Model file for the job. Use its own axes, mm. Face numbers are marked on the shaded views. A direction names the side the tool comes from. Give positions to 0.01 mm unless a question says otherwise; leave off trailing zeros. Loops run counter-clockwise (first coordinate to the right, second up) from the corner with the lowest first, then second, coordinate; pieces in that order, holes last. Notation, with made-up numbers: (36, -7.75) -> (65, -7.75) arc R28 cw to (65, 17.25) -> close; hole circle Ø9 at (-29, 17.5). An arc over 180 degrees is marked (long way). Use CSV: the item, a comma, the result in double quotes. Start each with the question number.
(1) 3-axis set-ups, long thin cutter, end or side, ignore diameter. For the marked faces 4, 5, 6 and 7: which of +Z, -Z, +X, -X, +Y, -Y reach the whole face in a straight line?
(2) Cut at B-B on z = 20. Write the cut outline in (x, y).
(3) Cut at A-A on y = -32. Write the cut outline in (x, z).
(4) Flat gauge pins, fed straight in: pin 1 (5 mm diameter, centred on y = 9.47, z = 25.63, fed in from +X); pin 2 (5.5 mm diameter, centred on y = -25, z = 22, fed in from -X); pin 3 (14 mm diameter, centred on x = 33, z = 13.5, fed in from +Y). Where does each tip first touch, or does it go through?
(5) Cut at D-D on y = 31.5. Write the cut outline in (x, z), then the cut area to 3 significant figures.
(6) Drill centre lines: probe 1 along Y at (x, z) = (-16, 24.5); probe 2 along X at (y, z) = (11, 22.5); probe 3 along Y at (x, z) = (30, 26.5). Where is each one in solid material? Low to high.
(7) Cut at C-C on x = -12. Write the cut outline in (y, z).
(8) Pull direction Y, two halves, no side cores. Call the marked faces 1, 2 and 3: pulls with the +Y half, pulls with the -Y half, needs draft (parallel to the pull), parting line crosses it, or undercut.
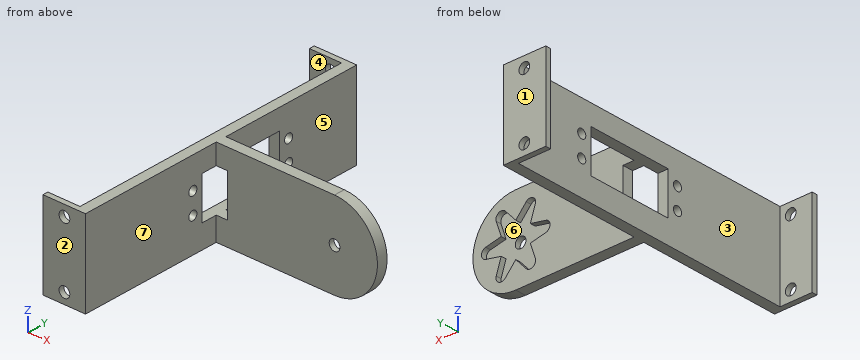
from build123d import *

# Parameters (mm, degrees)
BOSS_EXTRUDE2_DEPTH     = 40
FILLET3_RADIUS          = 20
FILLET3_LENGTH          = 5
SKETCH5_R               = 2.5
CUT_EXTRUDE2_DEPTH      = 40
SKETCH6_R               = 2.1
SKETCH6_W               = 19.7
SKETCH6_H               = 39.9
CUT_EXTRUDE3_DEPTH      = 10
CUT_EXTRUDE4_DEPTH      = 2.5
CUT_EXTRUDE5_DEPTH      = 138
CUT_EXTRUDE5_DEPTH_BACK = 49
SKETCH8_R               = 2.5


with BuildPart() as part:
    # Sketch4 → Boss-Extrude2 (new body)
    with BuildSketch(Plane.XY):
        Polygon((-19.701492537, 42.12238806), (-19.701492537, -27.87761194), (-19.701492537, -92.87761194), (-34.701492537, -92.87761194), (-34.701492537, -95.37761194), (-14.889132329, -95.37761194), (-14.889132329, -27.87761194), (60.298507463, -27.87761194), (60.298507463, -22.87761194), (-14.889132329, -22.87761194), (-14.889132329, 44.62238806), (-34.701492537, 44.62238806), (-34.701492537, 42.12238806), align=None)
    extrude(amount=BOSS_EXTRUDE2_DEPTH)

    # Fillet3: full round fillet: the end face becomes a half cylinder, R = half its width
    fillet3_face = Plane((60.298507463, -25.37761194, 20), x_dir=(0, 1, 0), z_dir=(1, 0, 0))  # on the end face: x along it, z out of the body
    fillet3_slab = fillet3_face.offset(-FILLET3_RADIUS / 2) * Box(FILLET3_LENGTH, 2 * FILLET3_RADIUS, FILLET3_RADIUS, mode=Mode.PRIVATE)  # the body's end, R deep
    fillet3_round = Plane((40.298507463, -25.37761194, 20), x_dir=(1, 0, 0), z_dir=(0, 1, 0)) * Cylinder(FILLET3_RADIUS, FILLET3_LENGTH, mode=Mode.PRIVATE)  # its axis R under the face
    add(fillet3_slab - fillet3_round, mode=Mode.SUBTRACT)

    # Sketch5 → Cut-Extrude2 (cut)
    with BuildSketch(Plane(origin=(0, -22.87761194, 0), x_dir=(1, 0, 0), z_dir=(0, 1, 0))):
        with Locations(Location((40.298507463, -20, 0), (0, 0, 270))):
            Circle(SKETCH5_R)
    extrude(amount=-CUT_EXTRUDE2_DEPTH, mode=Mode.SUBTRACT)

    # Sketch6 → Cut-Extrude3 (cut)
    with BuildSketch(Plane.ZY.offset(19.701492537)):
        with Locations(Location((15.780795158, 9.470750249, 0), (0, 0, 270))):
            Circle(SKETCH6_R)
        with Locations(Location((25.630795158, 9.470750249, 0), (0, 0, 270))):
            Circle(SKETCH6_R)
        with Locations(Location((15.780795158, -39.951540987, 0), (0, 0, 270))):
            Circle(SKETCH6_R)
        with Locations(Location((25.630795158, -39.951540987, 0), (0, 0, 270))):
            Circle(SKETCH6_R)
        with Locations((20.705795158, -15.240395369)):
            Rectangle(SKETCH6_W, SKETCH6_H)
    extrude(amount=-CUT_EXTRUDE3_DEPTH, mode=Mode.SUBTRACT)

    # Sketch7 → Cut-Extrude4 (cut)
    with BuildSketch(Plane(origin=(0, -22.87761194, 0), x_dir=(1, 0, 0), z_dir=(0, 1, 0))):
        with BuildLine():
            Line((35.419373283, -6.650386539), (40.298507463, -12.155040525))
            Line((40.298507463, -12.155040525), (45.177641643, -6.650386539))
            ThreePointArc((45.177641643, -6.650386539), (48.298507463, -6.143593539), (49.42004476, -9.099739121))
            Line((49.42004476, -9.099739121), (47.09244166, -16.077520262))
            Line((47.09244166, -16.077520262), (54.29917894, -17.550647418))
            ThreePointArc((54.29917894, -17.550647418), (56.298507463, -20), (54.29917894, -22.449352582))
            Line((54.29917894, -22.449352582), (47.09244166, -23.922479738))
            Line((47.09244166, -23.922479738), (49.42004476, -30.900260879))
            ThreePointArc((49.42004476, -30.900260879), (48.298507463, -33.856406461), (45.177641643, -33.349613461))
            Line((45.177641643, -33.349613461), (40.298507463, -27.844959475))
            Line((40.298507463, -27.844959475), (35.419373283, -33.349613461))
            ThreePointArc((35.419373283, -33.349613461), (32.298507463, -33.856406461), (31.176970165, -30.900260879))
            Line((31.176970165, -30.900260879), (33.504573265, -23.922479738))
            Line((33.504573265, -23.922479738), (26.297835985, -22.449352582))
            ThreePointArc((26.297835985, -22.449352582), (24.298507463, -20), (26.297835985, -17.550647418))
            Line((26.297835985, -17.550647418), (33.504573265, -16.077520262))
            Line((33.504573265, -16.077520262), (31.176970165, -9.099739121))
            ThreePointArc((31.176970165, -9.099739121), (32.298507463, -6.143593539), (35.419373283, -6.650386539))
        make_face()
    extrude(amount=-CUT_EXTRUDE4_DEPTH, mode=Mode.SUBTRACT)

    # Sketch8 → Cut-Extrude5 (cut, two sides: drawn at the far end of the back side and taken through both)
    with BuildSketch(Plane(origin=(0, 22.12238806, 0), x_dir=(-1, 0, 0), z_dir=(0, -1, 0)).offset(-CUT_EXTRUDE5_DEPTH_BACK)):
        with Locations(Location((24.701492537, -5, 0), (0, 0, 90))):
            Circle(SKETCH8_R)
        with Locations(Location((24.701492537, -35, 0), (0, 0, 90))):
            Circle(SKETCH8_R)
    extrude(amount=CUT_EXTRUDE5_DEPTH + CUT_EXTRUDE5_DEPTH_BACK, mode=Mode.SUBTRACT)


solid = part.part
Check result:
1,face 4,"+Z, -Z, -X"
1,face 5,"+Z, -Z, +X, +Y"
1,face 6,"+Y"
1,face 7,"+Z, -Z, +X, -Y"
2,outline,"(-34.7, -95.38) -> (-14.89, -95.38) -> (-14.89, -35.19) -> (-19.7, -35.19) -> (-19.7, -92.88) -> (-34.7, -92.88) -> close; (-34.7, 42.12) -> (-19.7, 42.12) -> (-19.7, 4.71) -> (-14.89, 4.71) -> (-14.89, 44.62) -> (-34.7, 44.62) -> close; (-9.7, -27.88) -> (37.8, -27.88) -> (37.8, -25.38) -> (24.3, -25.38) -> (24.3, -22.88) -> (-9.7, -22.88) -> close; (42.8, -27.88) -> (60.3, -27.88) -> (60.3, -22.88) -> (56.3, -22.88) -> (56.3, -25.38) -> (42.8, -25.38) -> close"
3,outline,"(-19.7, 0) -> (-14.89, 0) -> (-14.89, 10.86) -> (-19.7, 10.86) -> close; (-19.7, 30.56) -> (-14.89, 30.56) -> (-14.89, 40) -> (-19.7, 40) -> close"
4,pin 1,"x = -14.89"
4,pin 2,"x = -9.7"
4,pin 3,"y = -22.88"
5,outline,"(-19.7, 0) -> (-14.89, 0) -> (-14.89, 40) -> (-19.7, 40) -> close"
5,area,"192 mm²"
6,probe 1,"-95.38 to -41.72, -38.18 to -35.19, 4.71 to 7.7, 11.24 to 44.62"
6,probe 2,"-19.7 to -14.89"
6,probe 3,"-27.88 to -22.88"
7,outline,"(-27.88, 0) -> (-22.88, 0) -> (-22.88, 10.86) -> (-27.88, 10.86) -> close; (-27.88, 30.56) -> (-22.88, 30.56) -> (-22.88, 40) -> (-27.88, 40) -> close"
8,face 1,"pulls with the +Y half"
8,face 2,"pulls with the -Y half"
8,face 3,"undercut"
